from build123d import *

# Parameters (mm, degrees)
F0_W     = 50
F0_H     = 100
F1_DEPTH = 25
F2_T     = -10
F3_R     = 5


with BuildPart() as f1:
    # F0 (on Top) → F1 (new body)
    with BuildSketch(Plane.XY):
        with Locations((25, 50)):
            Rectangle(F0_W, F0_H)
    extrude(amount=F1_DEPTH)

    # F2
    f2_openings = [f1.faces().sort_by_distance(p)[0] for p in [
        (25, 50, 25),
    ]]
    offset(amount=F2_T, openings=f2_openings)

    # F3
    f3_edges = [f1.edges().sort_by_distance(p)[0] for p in [
        (10, 90, 17.5),
        (40, 90, 17.5),
        (40, 10, 17.5),
        (10, 10, 17.5),
    ]]
    fillet(f3_edges, radius=F3_R)


solid = f1.part
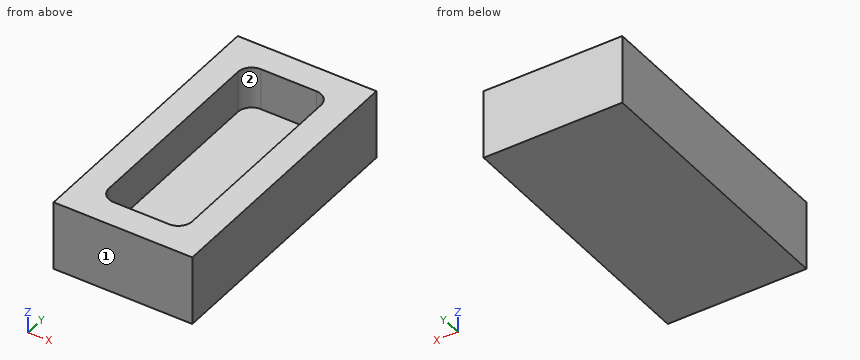
Input: part model. Units: mm. Frame: model coordinates. Face numbers are marked on the shaded views. A direction names the side the tool comes from. Coordinates: 2 decimals unless noted, no trailing zeros. Loops run counter-clockwise (first coordinate to the right, second up) from the corner with the lowest first, then second, coordinate; pieces in that order, holes last. Notation, with made-up numbers: (-7.5, 64.5) -> (48.5, 64.5) arc R19 cw to (48.5, 74.5) -> close; hole circle Ø10 at (57.5, -26). An arc over 180 degrees is marked (long way). Write item = value, one per line. Start each with the question number.
Item 1: First-contact query: P1, Ø15, axis at x = 23.5, y = 47, coming from the +Z side. Flat tip, straight axial feed; report the tip coordinate or a pass-through.
Item 2: Material intervals for line 1 (Y direction, x = 31.5, z = 11.5); line 2 (X direction, y = 62, z = 14); line 3 (Z direction, x = 19, y = 63), sorted ascending.
Item 3: Cut plane B-B, the plane y = 57. Return loops of the section in (x, z).
Item 4: Cut plane C-C, the plane x = 33. Return loops of the section in (y, z).
Item 5: Cut plane A-A, the plane z = 20.25. Return loops of the section in (x, y).
Item 6: Reachability of the marked faces 1 and 2 from +Z, -Z, +X, -X, +Y, -Y: full face, straight path, thin tool, end or side. Return the list, or none.
Ans:
q1.P1 = 10
q2.line_1 = 0 to 10, 90 to 100
q2.line_2 = 0 to 10, 40 to 50
q2.line_3 = 0 to 10
q3.outline = (0, 0) -> (50, 0) -> (50, 25) -> (40, 25) -> (40, 10) -> (10, 10) -> (10, 25) -> (0, 25) -> close
q4.outline = (0, 0) -> (100, 0) -> (100, 25) -> (90, 25) -> (90, 10) -> (10, 10) -> (10, 25) -> (0, 25) -> close
q5.outline = (0, 0) -> (50, 0) -> (50, 100) -> (0, 100) -> close; hole (10, 15) arc R5 ccw to (15, 10) -> (35, 10) arc R5 ccw to (40, 15) -> (40, 85) arc R5 ccw to (35, 90) -> (15, 90) arc R5 ccw to (10, 85) -> close
q6.face_1 = +Z, -Z, +X, -X, -Y
q6.face_2 = +Z
